Autodesk Inventor part; units mm, degrees
ref_plane "YZ Plane" through (0, 0, 0) normal (1, 0, 0) x (0, 1, 0)
ref_plane "XZ Plane" through (0, 0, 0) normal (0, 1, 0) x (-1, 0, 0)
ref_plane "XY Plane" through (0, 0, 0) normal (0, 0, 1) x (1, 0, 0)
sketch "Sketch1" plane through (0, 0, 0) normal (0, 0, 1) x (1, 0, 0)
  line L0 (-38, -3.2322) -> (38, -3.2322)
  line L1 (38, -3.2322) -> (38, 3.2322)
  line L2 (38, 3.2322) -> (9.4645, 31.7678)
  line L3 (9.4645, 31.7678) -> (-9.4645, 31.7678)
  line L4 (-9.4645, 31.7678) -> (-38, 3.2322)
  line L5 (-38, 3.2322) -> (-38, -3.2322)
  line L6 (-48, -3.2322) -> (48, -3.2322) construction
  line L7 (48, -3.2322) -> (0, 44.7678) construction
  line L8 (0, 44.7678) -> (-48, -3.2322) construction
  point P0 (0, 0)
  point P1 (0, -3.2322)
  point P2 (0, 31.7678)
  point P3 (38, 0)
  dimension "d0" = 76
  dimension "d1" = 96
  dimension "d2" = 2.5
  dimension "d3" = 35
extrude "Extrusion1" add sketch "Sketch1" along normal mid plane 0.6
sketch "Sketch4" plane through (0, 0, 0.3) normal (0, 0, 1) x (1, 0, 0)
  line L0 (-38, -3.2322) -> (38, -3.2322)
  line L1 (38, -3.2322) -> (38, 3.2322)
  line L2 (38, 3.2322) -> (9.4645, 31.7678)
  line L3 (9.4645, 31.7678) -> (-9.4645, 31.7678)
  line L4 (-9.4645, 31.7678) -> (-38, 3.2322)
  line L5 (-38, 3.2322) -> (-38, -3.2322)
  line L6 (-8.5, 30.2678) -> (8.5, 30.2678) construction
  point P0 (0, 0)
  point P1 (0, 30.2678)
  dimension "d19" = 17
  dimension "d20" = 33.5
hole "Hole1" at (-8.5, 30.2678, 0.3) at (8.5, 30.2678, 0.3) direction (0, 0, -1) diameter 1 end through all
fillet "Fillet1" radius 1 6 edges at (38, -3.2322, 0) (38, 3.2322, 0) (9.4645, 31.7678, 0) (-9.4645, 31.7678, 0) (-38, 3.2322, 0) (-38, -3.2322, 0)
properties part number "-ZPanel_PCBExtender" material "Epoxy Resin"
Check sheet for the modelled part. Datum: model origin and axes. Units: mm. Coordinates: 2 decimals unless noted, no trailing zeros. Order: outer loops, then holes, each group sorted by start corner. A loop starts at its lowest first (then second) coordinate and runs counter-clockwise, first axis right, second up. Notation, with made-up numbers: (-10.5, 38.25) -> (24.5, 38.25) arc R24 cw to (24.5, 53.25) -> close; hole circle Ø4 at (48, -0.75). An arc over 180 degrees is marked (long way). Write item = value, one per line. Start each with the question number.
1) Cross-section at B-B (x = -23.5). Enter the section's corners in (y, z), then the cut area to 3 significant figures.
2) Material ranges on L1, parallel to Y at x = 8.5, z = 0.15; L2, parallel to X at y = 5.5, z = -0.1; L3, parallel to X at y = 18.5, z = -0.2, recorded low to high.
3) Cross-section at C-C (y = 6). Enter the section's corners in (x, z), then the cut area to 3 significant figures.
4) Cross-section at A-A (z = -0.15). Enter the section's corners in (x, y), then the cut area to 3 significant figures.
Ans:
q1.outline = (-3.23, -0.3) -> (17.73, -0.3) -> (17.73, 0.3) -> (-3.23, 0.3) -> close
q1.area = 12.6 mm²
q2.L1 = -3.23 to 29.77, 30.77 to 31.77
q2.L2 = -35.73 to 35.73
q2.L3 = -22.73 to 22.73
q3.outline = (-35.23, -0.3) -> (35.23, -0.3) -> (35.23, 0.3) -> (-35.23, 0.3) -> close
q3.area = 42.3 mm²
q4.outline = (-38, -2.23) arc R1 ccw to (-37, -3.23) -> (37, -3.23) arc R1 ccw to (38, -2.23) -> (38, 2.82) arc R1 ccw to (37.71, 3.53) -> (9.76, 31.47) arc R1 ccw to (9.05, 31.77) -> (-9.05, 31.77) arc R1 ccw to (-9.76, 31.47) -> (-37.71, 3.53) arc R1 ccw to (-38, 2.82) -> close; hole circle Ø1 at (-8.5, 30.27); hole circle Ø1 at (8.5, 30.27)
q4.area = 1,840 mm²
